Print and shaded views of the part. All mm, measured from the part's lowest x, y and z. A direction names the side the tool comes from. Give positions to 0.01 mm unless a question says otherwise; leave off trailing zeros. Write each loop counter-clockwise with the first axis right and the second up, starting at its lowest first coordinate (ties: lowest second). Pieces come first, ordered by that corner, then holes.
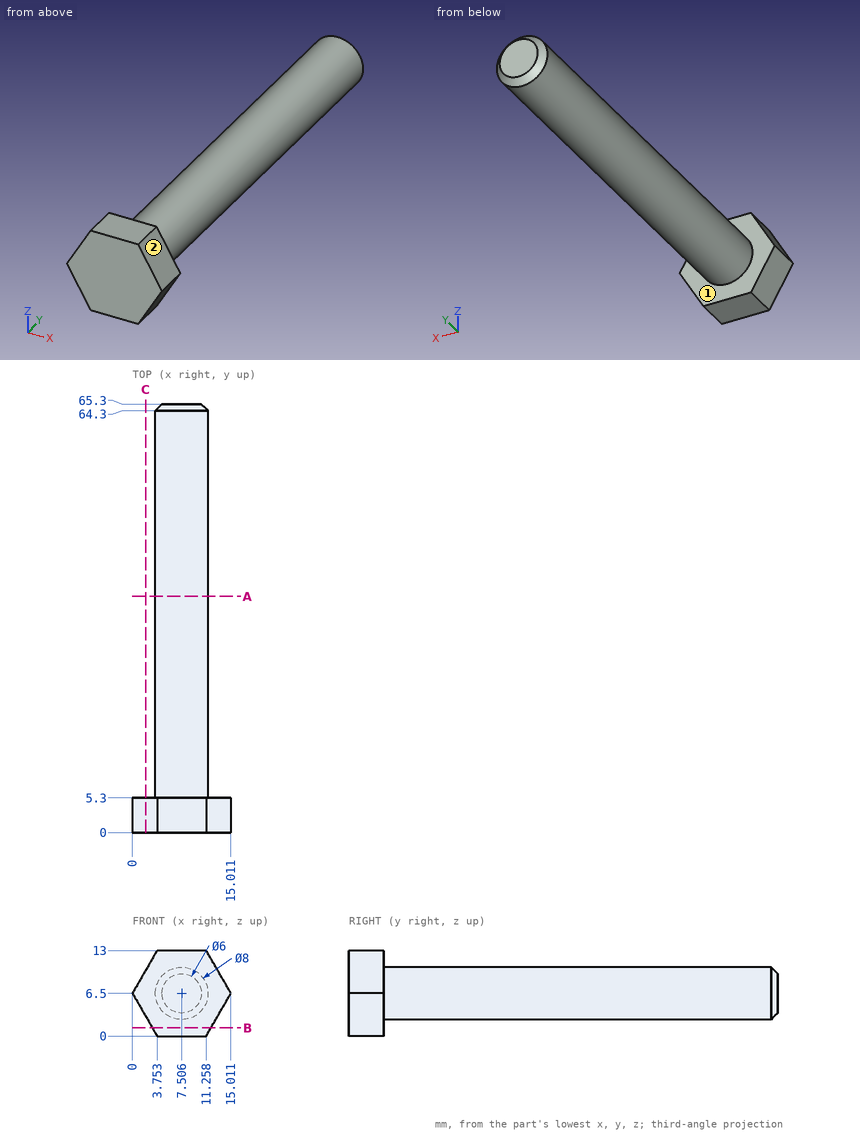
1. Saw through at A-A on y = 36. Give the cut face in (x, z) (1 decimal).
2. Saw through at B-B on z = 1.25. Give the cut face in (x, y).
3. Saw through at C-C on x = 2. Give the cut face in (y, z) (1 decimal).
4. Drop flat-ended pins along their axis: pin 1 (5 mm diameter, centred on y = 48, z = 10.5, fed in from +X); pin 2 (3 mm diameter, centred on y = 57, z = 2, fed in from +X); pin 3 (8 mm diameter, centred on x = 6, y = 47.5, fed in from -Z). Give the stop position or say it passes through.
5. Drill centre lines: line 1 along Y through (x, z) = (8.25, 2.25); line 2 along X through (y, z) = (44.5, 6.75); line 3 along Z through (x, y) = (8.25, 40). Where is each one in solid material? Low to high.
6. 3-axis set-ups, long thin cutter, end or side, ignore diameter. For the marked faces 1 and 2: which of +Z, -Z, +X, -X, +Y, -Y reach the whole face in a straight line?
Outcome:
1. outline: circle Ø8 at (7.5, 6.5)
2. outline: (3.03, 0) - (11.98, 0) - (11.98, 5.3) - (3.03, 5.3) - close
3. outline: (0, 3) - (5.3, 3) - (5.3, 10) - (0, 10) - close
4. pin 1: stops at x = 11.21
4. pin 2: stops at x = 10.15
4. pin 3: stops at z = 2.5
5. line 1: y = 0 to 5.3
5. line 2: x = 3.51 to 11.5
5. line 3: z = 2.57 to 10.43
6. face 1: +Y
6. face 2: +Z, +X, +Y, -Y
